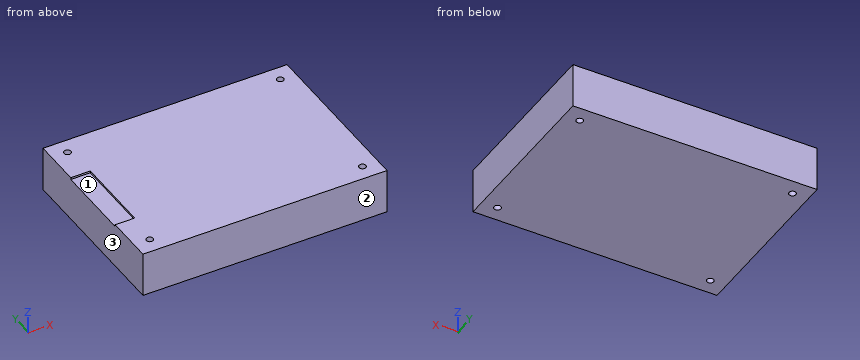
Solid Edge part; units mm, degrees
sketch "Sketch1" plane through (0, 0, 0) normal (0, 0, 1) x (1, 0, 0)
  line L0 (0, 0) -> (125, 0)
  line L1 (125, 0) -> (125, 90)
  line L2 (125, 90) -> (0, 90)
  line L3 (0, 90) -> (0, 0)
  dimension "D1" = 125
  dimension "D2" = 0
extrude "Protrusion1" add sketch "Sketch1" along normal blind 23
hole "Bohrung_1" at (8, 82, 23) direction (0, 0, -1) diameter 3.5 end through all
hole "Hole1" at (117, 82, 23) direction (0, 0, -1) diameter 3.5 end through all
hole "Hole2" at (8, 8, 23) direction (0, 0, -1) diameter 3.5 end through all
hole "Hole3" at (117, 8, 23) direction (0, 0, -1) diameter 3.5 end through all
sketch "Sketch2" plane through (62.5, 45, 23) normal (0, 0, 1) x (1, 0, 0)
  line L0 (-62.5, 20) -> (-52.5, 20)
  line L1 (-52.5, 20) -> (-52.5, -20)
  line L2 (-52.5, -20) -> (-62.5, -20)
  line L3 (-62.5, -20) -> (-62.5, 20)
  dimension "D1" = 62.5
  dimension "D2" = 62.5
extrude "Cutout1" cut sketch "Sketch2" against normal blind 1
properties material "Elektronik"
CAD build for the part. Positions are in the model's coordinates, mm. Face numbers are marked on the shaded views. Round coordinates to 2 decimals unless told otherwise and drop trailing zeros. Write each loop counter-clockwise with the first axis right and the second up, starting at its lowest first coordinate (ties: lowest second). Pieces come first, ordered by that corner, then holes. Notation, with made-up numbers: M 80,-13.5 L 114,-13.5 A26 cw 114,20.5 Z; hole C 40.25,-34.75 d2. An arc over 180 degrees is marked long. Put each result on its own line as item: value. Start each with the question number.
1) Pull direction Y, two halves, no side cores. Call the marked faces 1, 2 and 3: pulls with the +Y half, pulls with the -Y half, needs draft (parallel to the pull), parting line crosses it, or undercut.
2) Saw through at B-B, the plane y = 8. Write the cut outline in (x, z), and give its area (3 significant figures).
3) Drill centre lines: probe 1 along X at (y, z) = (82, 10); probe 2 along Y at (x, z) = (8, 12); probe 3 along X at (y, z) = (6.5, 16.5). Where is each one in solid material? Low to high. Write a range as [from, to].
4) Saw through at A-A, the plane x = 8. Write the cut outline in (y, z), and give its area (3 significant figures).
5) Pin check, flat tip, straight feed: pin 1 Ø5 at (x, y) = (2.5, 37.5) entering from +Z. Stop position of the tip, or through.
6) Saw through at C-C, the plane x = 117. Write the cut outline in (y, z), and give its area (3 significant figures).
Resolved:
1. face 1: undercut
1. face 2: pulls with the -Y half
1. face 3: needs draft
2. outline: M 0,0 L 6.25,0 L 6.25,23 L 0,23 Z; M 9.75,0 L 115.25,0 L 115.25,23 L 9.75,23 Z; M 118.75,0 L 125,0 L 125,23 L 118.75,23 Z
2. area: 2,710 mm²
3. probe 1: [0, 6.25], [9.75, 115.25], [118.75, 125]
3. probe 2: [0, 6.25], [9.75, 80.25], [83.75, 90]
3. probe 3: [0, 7.1], [8.9, 116.1], [117.9, 125]
4. outline: M 0,0 L 6.25,0 L 6.25,23 L 0,23 Z; M 9.75,0 L 80.25,0 L 80.25,23 L 65,23 L 65,22 L 25,22 L 25,23 L 9.75,23 Z; M 83.75,0 L 90,0 L 90,23 L 83.75,23 Z
4. area: 1,870 mm²
5. pin 1: z = 22
6. outline: M 0,0 L 6.25,0 L 6.25,23 L 0,23 Z; M 9.75,0 L 80.25,0 L 80.25,23 L 9.75,23 Z; M 83.75,0 L 90,0 L 90,23 L 83.75,23 Z
6. area: 1,910 mm²
